from build123d import *

# Parameters (mm, degrees)
SKETCH1_R           = 2.5
BOSS_EXTRUDE1_DEPTH = 6
SKETCH2_R           = 2.95
BOSS_EXTRUDE2_DEPTH = 1
DOME1_FACE_RADIUS   = 2.5
DOME1_HEIGHT        = 2.6
CUT_EXTRUDE1_REACH  = 10.6
SKETCH3_W           = 4.756042082
SKETCH3_H           = 0.515985698
SKETCH4_W           = 0.5
SKETCH4_H           = 0.5
BOSS_EXTRUDE3_DEPTH = 4


with BuildPart() as part:
    # Sketch1 → Boss-Extrude1 (new body)
    with BuildSketch(Plane(origin=(0, 0, 0), x_dir=(1, 0, 0), z_dir=(0, 1, 0))):
        Circle(SKETCH1_R)
    extrude(amount=BOSS_EXTRUDE1_DEPTH)

    # Sketch2 → Boss-Extrude2 (add)
    with BuildSketch(Plane(origin=(0, 0, 0), x_dir=(1, 0, 0), z_dir=(0, 1, 0))):
        Circle(SKETCH2_R)
    extrude(amount=BOSS_EXTRUDE2_DEPTH)

    # Dome1: a dome of height H over a round flat face of radius A is a cap of a sphere of radius (A * A + H * H) / (2 * H)
    dome1_r = (DOME1_FACE_RADIUS * DOME1_FACE_RADIUS + DOME1_HEIGHT * DOME1_HEIGHT) / (2 * DOME1_HEIGHT)
    dome1_base = Plane((0, 6, 0), z_dir=(0, 1, 0))
    with Locations(dome1_base.offset(DOME1_HEIGHT - dome1_r)):
        dome1_ball = Sphere(dome1_r, mode=Mode.PRIVATE)
    add(split(dome1_ball, bisect_by=dome1_base, keep=Keep.TOP, mode=Mode.PRIVATE))

    # Sketch3 → Cut-Extrude1 (cut, up to next)
    with BuildSketch(Plane.XZ, mode=Mode.PRIVATE) as cut_extrude1_sk1:
        with Locations((0.213124527, 2.757992849)):
            Rectangle(SKETCH3_W, SKETCH3_H)
    cut_extrude1_tool1 = extrude(cut_extrude1_sk1.sketch, amount=-CUT_EXTRUDE1_REACH, mode=Mode.PRIVATE) & part.part
    add(cut_extrude1_tool1.solids().sort_by_distance((0.213125, 0, 2.757993))[0], mode=Mode.SUBTRACT)

    # Sketch4 → Boss-Extrude3 (add)
    with BuildSketch(Plane.XZ):
        with Locations((0, 1.905)):
            Rectangle(SKETCH4_W, SKETCH4_H)
        with Locations((0, 0.635)):
            Rectangle(SKETCH4_W, SKETCH4_H)
        with Locations((0, -0.635)):
            Rectangle(SKETCH4_W, SKETCH4_H)
        with Locations((0, -1.905)):
            Rectangle(SKETCH4_W, SKETCH4_H)
    extrude(amount=BOSS_EXTRUDE3_DEPTH)


solid = part.part
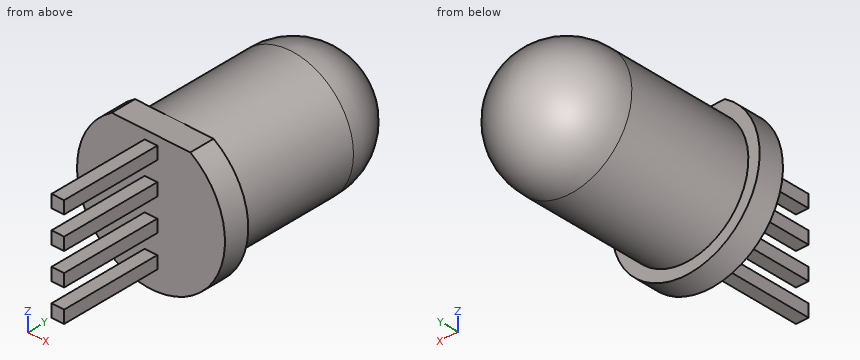
Can you work these out from the model? Positions are in its coordinate system, mm. Coordinates: 2 decimals unless noted, no trailing zeros. Write each loop counter-clockwise with the first axis right and the second up, starting at its lowest first coordinate (ties: lowest second). Pieces come first, ordered by that corner, then holes. Notation, with made-up numbers: M 70.5,79.25 L 78.5,79.25 A24 ccw 78.5,98.25 Z; hole C 33,75.25 d9. An arc over 180 degrees is marked long. Use one line per item in the form item = value.
Q1. If we section it at B-B (x = -1.75): Write out the boundary of the cut face in (y, z).
Model answer:
outline = M 0,-2.37 L 1,-2.37 L 1,-1.79 L 6,-1.79 A1.79 ccw long 6,1.79 L 1,1.79 L 1,2.37 L 0,2.37 Z
Q2. I need wall thicknesses on line 1 along X through (y, z) = (-1, 0.7); line 2 along Z through (x, y) = (0, 6.25); line 3 along Y through (x, z) = (1.75, -2.15). Which ranges of each line are inside material? Lowest first, please. Write a range as from..to.
Model answer:
line_1 = -0.25..0.25
line_2 = -2.5..2.5
line_3 = 0..1
Q3. For P1, Ø0.6, axis at x = 0, y = -1.5, coming from the -Z side (3 decimals); P2, Ø1.5, axis at x = -0.5, y = 4, coming from the +Z side; P3, Ø0.6, axis at y = -2, z = 0.5, coming from the +X side; P4, Ø0.6, axis at x = 0, y = -2, coming from the +Z side (3 decimals), each with a flat end and sliding along its axis, tell me the tip position at first contact or that it passes through.
Model answer:
P1 = -2.155
P2 = 2.5
P3 = 0.25
P4 = 2.155
Q4. If we section it at C-C (y = 5): Write out the boundary of the cut face in (x, z), then the cut area to 3 significant figures.
Model answer:
outline = C 0,0 d5
area = 19.6 mm^2
